Read the model definition and answer for the solid it produces. Units are mm, in the model's axes. Face numbers are marked on the shaded views. A direction names the side the tool comes from. Round coordinates to 2 decimals unless told otherwise and drop trailing zeros. Order: outer loops, then holes, each group sorted by start corner. A loop starts at its lowest first (then second) coordinate and runs counter-clockwise, first axis right, second up. Notation, with made-up numbers: (44.5, 87) -> (101.5, 87) arc R21 ccw to (101.5, 91) -> close; hole circle Ø1 at (51.25, 73.25). An arc over 180 degrees is marked (long way). Use a Markdown table: item, result. Add a question column.
1. The mould has two halves that part along X. Classify the marked faces 1, 2 and 3: +X half, -X half, draft (parallel to the pull), parting line (faces both ways), or undercut.
2. Consider L1, parallel to Y at x = 5, z = -1.6; L2, parallel to X at y = -5.5, z = -0.8; L3, parallel to Z at x = 8.5, y = 1.5. Determine where each line is inside the solid, lowest interval first. Write a range as [from, to].
3. Section A-A, the plane y = 0 is taken. Give the number of separate pieces and of enclosed holes in the cut face, then the cut area to 3 significant figures.
4. Section D-D, the plane y = 5 is taken. Give the vertices of the cut face in (x, z), then the cut area to 4 significant figures.
5. Section C-C, the plane x = 7.75 is taken. Give the vertices of the cut face in (y, z), then the cut area to 3 significant figures.
6. Given pin 1 (1 mm diameter, centred on x = -2.5, z = -1.5, fed in from +Y); pin 2 (1.2 mm diameter, centred on x = 4.91, y = 4.99, fed in from -Z); pin 3 (2.5 mm diameter, centred on x = 0.06, y = -7, fed in from -Z); pin 4 (1 mm diameter, centred on x = 4.5, z = -1, fed in from +Y), each flat-ended and moving along its own axis, determine where each tip first touches the part or whether it passes through.
7. For the marked faces 4, 5 and 6, determine the directions among +Z, -Z, +X, -X, +Y, -Y from which every point of the face is accessible in a straight line to the end or side of a thin tool.
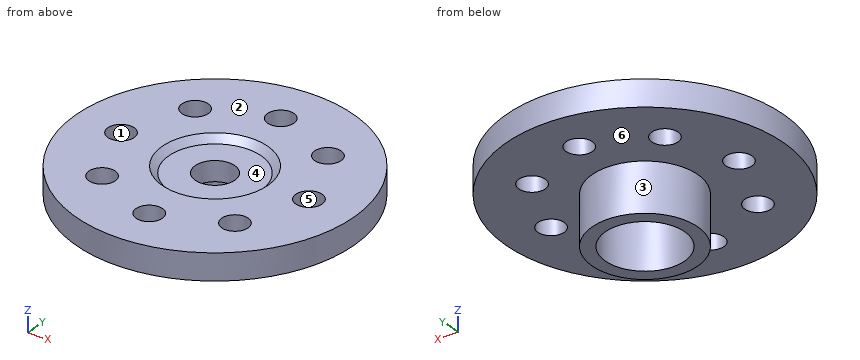
Autodesk Inventor part; units mm, degrees
ref_plane "YZ Plane" through (0, 0, 0) normal (1, 0, 0) x (0, 1, 0)
ref_plane "XZ Plane" through (0, 0, 0) normal (0, 1, 0) x (-1, 0, 0)
ref_plane "XY Plane" through (0, 0, 0) normal (0, 0, 1) x (1, 0, 0)
sketch "スケッチ1" plane through (0, 0, 0) normal (0, 0, 1) x (1, 0, 0)
  circle A0 centre (0, 0) radius 10.5
  circle A1 centre (0, 0) radius 3.5
  circle A2 centre (0, 0) radius 7 construction
  circle A3 centre (0, 0) radius 7 construction
  circle A4 centre (0, 0) radius 7 construction
  circle A5 centre (0, 0) radius 7 construction
  circle A6 centre (0, 0) radius 7 construction
  circle A7 centre (0, 0) radius 7 construction
  circle A8 centre (0, 0) radius 7 construction
  circle A9 centre (0, 0) radius 7 construction
  circle A10 centre (0, 0) radius 4
  circle A11 centre (0, 0) radius 1.5
  circle A12 centre (0, 0) radius 3
  point P0 (-0.061, 6.9997)
  point P1 (-4.9927, 4.9064)
  point P2 (-6.9997, -0.061)
  point P3 (-4.9064, -4.9927)
  point P4 (0.061, -6.9997)
  point P5 (4.9927, -4.9064)
  point P6 (6.9997, 0.061)
  point P7 (4.9064, 4.9927)
  dimension "d2" = 14
  dimension "d0" = 21
  dimension "d1" = 7
  dimension "d5" = 360
  dimension "d7" = 8
  dimension "d8" = 3
  dimension "d11" = 6
extrude "押し出し1" add sketch "スケッチ1" against normal blind 2 contours A0 | A1 | A10 | A12
extrude "押し出し2" add sketch "スケッチ1" against normal blind 5.7 contours A1 | A10
extrude "押し出し3" cut sketch "スケッチ1" against normal blind 0.5 contours A1 | A12
chamfer "面取り1" distance 0.5 angle 45 1 edges at (-3.5, 0, 0)
hole "穴1" at (-0.061, 6.9997, 0) at (-4.9927, 4.9064, 0) at (-6.9997, -0.061, 0) at (-4.9064, -4.9927, 0) at (0.061, -6.9997, 0) at (4.9927, -4.9064, 0) at (6.9997, 0.061, 0) at (4.9064, 4.9927, 0) direction (0, 0, -1) diameter 2 end through all
sketch "スケッチ2" plane through (0, 0, 0) normal (0, 0, 1) x (1, 0, 0)
  circle A0 centre (4.9064, 4.9927) radius 1
  circle A1 centre (6.9997, 0.061) radius 1
  circle A2 centre (4.9927, -4.9064) radius 1
  circle A3 centre (0.061, -6.9997) radius 1
  circle A4 centre (-4.9064, -4.9927) radius 1
  circle A5 centre (-6.9997, -0.061) radius 1
  circle A6 centre (-4.9927, 4.9064) radius 1
  circle A7 centre (-0.061, 6.9997) radius 1
  circle A8 centre (0, 0) radius 10.5
  circle A9 centre (0, 0) radius 4
  circle A10 centre (0, 0) radius 8
  circle A11 centre (-0.061, 6.9997) radius 1
  dimension "d26" = 16
properties part number "servohorn_zegi" material "アルミニウム 6061-AHC"
Verdict:
| question | item | result |
|---|---|---|
| 1 | face 1 | undercut |
| 1 | face 2 | draft |
| 1 | face 3 | parting line |
| 2 | L1 | y = [-9.23, -5.91], [-3.91, 4], [5.99, 9.23] |
| 2 | L2 | x = [-8.94, -5.77], [-4.04, 4.19], [5.8, 8.94] |
| 2 | L3 | z = [-2, 0] |
| 3 | separate pieces | 4 |
| 3 | enclosed holes | 0 |
| 3 | area | 33.2 mm2 |
| 4 | outline | (-9.23, -2) -> (-5.99, -2) -> (-5.99, 0) -> (-9.23, 0) -> close; (-4, -2) -> (3.91, -2) -> (3.91, 0) -> (-4, 0) -> close; (5.91, -2) -> (9.23, -2) -> (9.23, 0) -> (5.91, 0) -> close |
| 4 | area | 28.95 mm2 |
| 5 | outline | (-7.08, -2) -> (-0.6, -2) -> (-0.6, 0) -> (-7.08, 0) -> close; (0.72, -2) -> (7.08, -2) -> (7.08, 0) -> (0.72, 0) -> close |
| 5 | area | 25.7 mm2 |
| 6 | pin 1 | stops at y = 10.31 |
| 6 | pin 2 | passes through |
| 6 | pin 3 | stops at z = -2 |
| 6 | pin 4 | stops at y = 9.71 |
| 7 | face 4 | +Z |
| 7 | face 5 | +Z, -Z |
| 7 | face 6 | -Z |
